from build123d import *

# Parameters (mm, degrees)
F0_W      = 21.5
F0_H      = 30
F1_DEPTH  = 5
F3_DEPTH  = 108
F4_R      = 2
F5_DEPTH  = 25
F7_R      = 5
F6_W      = 8
F6_H      = 16
F6_W_2    = 2.5
F6_W_3    = 3
F8_DEPTH  = 20
F9_R      = 7.99999
F10_R     = 3
F11_DEPTH = 40
F12_W     = 80
F12_H     = 50
F13_DEPTH = 25
F15_DEPTH = 15
F16_R     = 5
F17_R     = 1.75
F18_DEPTH = 25


# Not quite as in the source:
# - a fillet or chamfer is up to 0.001 mm smaller than in the source, because OpenCascade refuses the exact size


with BuildPart() as f1:
    # F0 (on Top) → F1 (new body)
    with BuildSketch(Plane.XY):
        with Locations((-43.25, 15)):
            Rectangle(F0_W, F0_H)
        Polygon((-32.5, 0), (-54, 0), (-54, -20), (54, -20), (54, 0), (32.5, 0), align=None)
        with Locations((43.25, 15)):
            Rectangle(F0_W, F0_H)
    extrude(amount=F1_DEPTH)

    # F2 (on face) → F3 (join)
    with BuildSketch(Plane(origin=(-54, 0, 0), x_dir=(0, -1, 0), z_dir=(-1, 0, 0))):
        Polygon((20, 5), (20, 0), (54.3258497444, -83.6021589144), (57.101034605, -82.4627077355), (21.1900987758, 5), align=None)
    extrude(amount=-F3_DEPTH)

    # F4 (on face) → F5 (cut)
    with BuildSketch(Plane(origin=(0, -19.8899648845, 8.1665348708), x_dir=(1, 0, 0), z_dir=(0, -0.9250616202, 0.3798170597))):
        with Locations((-43.5, -83.4230529098)):
            Circle(F4_R)
        with Locations((43.5, -83.4230529098)):
            Circle(F4_R)
    extrude(amount=-F5_DEPTH, mode=Mode.SUBTRACT)

    # F7
    f7_edges = [f1.edges().sort_by_distance(p)[0] for p in [
        (0, -21.190099, 5),
        (0, -20, 0),
        (-54, 30, 2.5),
        (54, 30, 2.5),
        (54, -55.713442, -83.032433),
        (-54, -55.713442, -83.032433),
        (-32.5, 0, 2.5),
        (32.5, 0, 2.5),
    ]]
    fillet(f7_edges, radius=F7_R)

    # F6 (on face) → F8 (join)
    with BuildSketch(Plane.XY.offset(5)):
        with Locations((-8.45, -8)):
            Rectangle(F6_W, F6_H)
        with Locations((0.1, -8)):
            Rectangle(F6_W_2, F6_H)
        with Locations((6.15, -8)):
            Rectangle(F6_W_3, F6_H)
    extrude(amount=F8_DEPTH)

    # F9 (radius 8 in the source; OpenCascade refuses exactly that, so slightly less here)
    f9_edges = [f1.edges().sort_by_distance(p)[0] for p in [
        (-8.45, -16, 25),
        (0.1, -16, 25),
        (6.15, -16, 25),
        (-8.45, 0, 25),
        (0.1, 0, 25),
        (6.15, 0, 25),
    ]]
    fillet(f9_edges, radius=F9_R)

    # F10 (on face) → F11 (cut)
    with BuildSketch(Plane.YZ.offset(7.65)):
        with Locations((-8, 17)):
            Circle(F10_R)
    extrude(amount=-F11_DEPTH, mode=Mode.SUBTRACT)

    # F12 (on face) → F13 (cut)
    with BuildSketch(Plane(origin=(0, -19.8899648845, 8.1665348708), x_dir=(1, 0, 0), z_dir=(0, -0.9250616202, 0.3798170597))):
        with Locations((0, -41.7751698217)):
            Rectangle(F12_W, F12_H)
    extrude(amount=-F13_DEPTH, mode=Mode.SUBTRACT)

    # F14 (on face) → F15 (join)
    with BuildSketch(Plane(origin=(0, 0, 0), x_dir=(1, 0, 0), z_dir=(0, 0, -1))):
        Polygon((-54, 5), (-54, 0), (-27.5, 0), (27.5, 0), (54, 0), (54, 5), align=None)
    extrude(amount=F15_DEPTH)

    # F16
    f16_edges = [f1.edges().sort_by_distance(p)[0] for p in [
        (54, -2.5, -15),
        (-54, -2.5, -15),
    ]]
    fillet(f16_edges, radius=F16_R)

    # F17 (on face) → F18 (cut)
    with BuildSketch(Plane.XY.offset(5)):
        with Locations((-43.6119101942, 20)):
            Circle(F17_R)
        with Locations((43.6119101942, 20)):
            Circle(F17_R)
    extrude(amount=-F18_DEPTH, mode=Mode.SUBTRACT)


solid = f1.part
Could you check a few things on this model? Use its own coordinates, in mm. A direction names the side the tool comes from. Give positions to 0.01 mm unless a question says otherwise; leave off trailing zeros. Order: outer loops, then holes, each group sorted by start corner. A loop starts at its lowest first (then second) coordinate and runs counter-clockwise, first axis right, second up. Notation, with made-up numbers: (-14, -9.5) - (35, -9.5) arc R10 ccw to (35, -5.5) - close; hole circle Ø7 at (-6, 59.5). An arc over 180 degrees is marked (long way). One line per question, with ' | ' between items. Start each with the question number.
Item 1: I want a section at B-B on z = 10. Write out the boundary of the cut face in (x, y), then the cut area to 3 significant figures.
Item 2: I need wall thicknesses on probe 1 along Z at (x, y) = (-43.5, 24.5); probe 2 along Z at (x, y) = (6.4, -8); probe 3 along Y at (x, z) = (-27, -10.5). Which ranges of each line are inside material? Lowest first, please. Write a range as [from, to].
Item 3: I want a section at A-A on y = 13.5. Write out the boundary of the cut face in (x, z), then the cut area to 3 significant figures.
Item 4: I want a section at D-D on z = -18.5. Write out the boundary of the cut face in (x, y).
Item 5: Thinking about a two-plate mould opening in Z: for faces 1 (the cylindrical face through (6.17, -8.65, 14.07)), 2 (the flat face through (1, -5, -7)), 3 (the flat face through (-0.756, -44.913, -60.677)), which applies, pulls with the +Z half, pulls with the -Z half, needs draft (parallel to the pull), parting line crosses it, or undercut?
Item 6: I want a section at C-C on x = 24. Write out the boundary of the cut face in (y, z), then the cut area to 3 significant figures.
Item 7: I'm going to push flat-ended pins straight in: pin 1 Ø1.5 at (x, y) = (5, -11) entering from -Z; pin 2 Ø4 at (x, z) = (36.5, -9) entering from -Y; pin 3 Ø5 at (y, z) = (-8, 14) entering from -X. Where does each tip first touch, or does it pass through?
Item 8: For faces 4 (the flat face through (-12.45, -8, 13)), 5 (the cylindrical face through (31.07, 1.5, 2.54)), 6 (the flat face through (-44, 15, 0)), 7 (the cylindrical face through (52, -3, -14)), which set-ups out of +Z, -Z, +X, -X, +Y, -Y let a thin tool reach every point of the face, with its end or its side?
Verdict:
1) outline: (-12.45, -16) - (-4.45, -16) - (-4.45, 0) - (-12.45, 0) - close; (-1.15, -16) - (1.35, -16) - (1.35, 0) - (-1.15, 0) - close; (4.65, -16) - (7.65, -16) - (7.65, 0) - (4.65, 0) - close | area: 216 mm^2
2) probe 1: [0, 5] | probe 2: [0, 14], [20, 25] | probe 3: [-5, 0]
3) outline: (-54, 0) - (-32.5, 0) - (-32.5, 5) - (-54, 5) - close; (32.5, 0) - (54, 0) - (54, 5) - (32.5, 5) - close | area: 215 mm^2
4) outline: (-54, -30.84) - (-40, -30.84) - (-40, -27.6) - (-54, -27.6) - close; (40, -30.84) - (54, -30.84) - (54, -27.6) - (40, -27.6) - close
5) face 1: undercut | face 2: needs draft | face 3: pulls with the -Z half
6) outline: (-57.1, -82.46) - (-54.33, -83.6) - (-42.48, -54.74) - (-45.25, -53.6) - close; (-26.26, -7.35) - (-23.49, -8.49) - (-21.27, -3.1) arc R5 cw to (-16.65, 0) - (-5, 0) - (-5, -15) - (0, -15) - (0, 5) - (-17.84, 5) arc R5 ccw to (-22.46, 1.9) - close | area: 305 mm^2
7) pin 1: z = 0 | pin 2: y = -26.26 | pin 3: x = -12.45
8) face 4: +Z, -X, +Y, -Y | face 5: +Z, -Z, +Y | face 6: -Z, +X, -X, +Y | face 7: -Z, +X, +Y
